The listing builds one solid part. Answer for the finished solid, in the listing's coordinates (mm). A direction names the side the tool comes from. Coordinates: 2 decimals unless noted, no trailing zeros. Write each loop counter-clockwise with the first axis right and the second up, starting at its lowest first coordinate (ties: lowest second). Pieces come first, ordered by that corner, then holes.
from build123d import *

# Parameters (mm, degrees)
SKETCH1_R           = 3.5
SKETCH1_R_2         = 1.8
BOSS_EXTRUDE1_DEPTH = 12
BOSS_EXTRUDE2_DEPTH = 1.5
BOSS_EXTRUDE3_DEPTH = 1.5
CUT_EXTRUDE1_DEPTH  = 5
SKETCH6_R           = 2.75
CUT_EXTRUDE2_DEPTH  = 6
FILLET1_R           = 0.5


with BuildPart() as part:
    # Sketch1 → Boss-Extrude1 (new body)
    with BuildSketch(Plane.XY):
        Circle(SKETCH1_R)
        Circle(SKETCH1_R_2, mode=Mode.SUBTRACT)
    extrude(amount=BOSS_EXTRUDE1_DEPTH)

    # Sketch2 → Boss-Extrude2 (add, symmetric)
    with BuildSketch(Plane(origin=(0, 0, 0), x_dir=(1, 0, 0), z_dir=(0, 1, 0))):
        with BuildLine():
            Line((-5, -17), (-5, -12))
            Line((-5, -12), (5, -12))
            Line((5, -12), (5, -17))
            ThreePointArc((5, -17), (0, -22), (-5, -17))
        make_face()
    extrude(amount=BOSS_EXTRUDE2_DEPTH, both=True)

    # Sketch3 → Boss-Extrude3 (add, symmetric)
    with BuildSketch(Plane(origin=(0, 0, 0), x_dir=(1, 0, 0), z_dir=(0, 1, 0))):
        Polygon((5, -12), (0, -3.339745962), (-5, -12), align=None)
    extrude(amount=BOSS_EXTRUDE3_DEPTH, both=True)

    # Sketch5 → Cut-Extrude1 (cut, symmetric)
    with BuildSketch(Plane(origin=(0, 0, 0), x_dir=(0, 0, -1), z_dir=(1, 0, 0))):
        Polygon((-12, 1.5), (-4, 3.5), (-12, 3.5), align=None)
    cut_extrude1 = extrude(amount=CUT_EXTRUDE1_DEPTH, both=True, mode=Mode.SUBTRACT)

    # Mirror1: Cut-Extrude1 across plane
    add(cut_extrude1.mirror(Plane.ZX), mode=Mode.SUBTRACT)

    # Sketch6 → Cut-Extrude2 (cut, through all)
    with BuildSketch(Plane(origin=(0, 1.5, 0), x_dir=(1, 0, 0), z_dir=(0, 1, 0))):
        with Locations((0, -17)):
            Circle(SKETCH6_R)
    extrude(amount=-CUT_EXTRUDE2_DEPTH, mode=Mode.SUBTRACT)

    # Fillet1
    fillet1_edges = [part.edges().sort_by_distance(p)[0] for p in [
        (-5, -1.5, 14.5),
        (0, -1.5, 22),
        (-5, 1.5, 14.5),
        (5, 1.5, 14.5),
        (-2.342808298, 2.600240235, 7.599039061),
        (2.342808298, -2.600240235, 7.599039061),
        (-4.08113883, 1.5, 10.408485769),
        (-4.08113883, -1.5, 10.408485769),
        (5, -1.5, 14.5),
        (-2.75, -1.5, 17),
        (-2.75, 1.5, 17),
        (4.08113883, 1.5, 10.408485769),
        (0, 1.5, 22),
    ]]
    fillet(fillet1_edges, radius=FILLET1_R)


solid = part.part
1. Flat-ended cylindrical pins translate along their axes: P1, Ø1.5, axis at x = 1, z = 19, coming from the -Y side; P2, Ø4, axis at x = 2.5, y = -2.5, coming from the +Z side; P3, Ø1.5, axis at y = -0.5, z = 2.5, coming from the +X side. Find the tip coordinate at first contact, or state that the pin passes through.
Results found:
P1: stops at y = -1.42
P2: stops at z = 21.87
P3: stops at x = 3.5
2. A tool of negligible diameter and unlimited length cuts with its end or side. For faces 4 (the cylindrical face through (-3.497, 0.154, 4.123)), 5 (the cylindrical face through (4.027, 1.35, 10.599)), from which of +Z, -Z, +X, -X, +Y, -Y can it reach the whole face along a straight path? Write none if from no direction.
Results found:
face 4: -Z
face 5: -Z, +X, +Y
3. Section A-A on y = 0 is taken. Give the vertices of the cut face in (x, z).
Results found:
outline: (-5, 12) - (-3.5, 9.4) - (-3.5, 0) - (-1.8, 0) - (-1.8, 6.46) - (0, 3.34) - (1.8, 6.46) - (1.8, 0) - (3.5, 0) - (3.5, 9.4) - (5, 12) - (5, 17) arc R5 ccw to (-5, 17) - close; hole circle Ø5.5 at (0, 17)
4. Section C-C on z = 8.25 is taken. State how many separate pieces and enclosed holes the cut face has, then the cut area to 3 significant figures.
Results found:
separate pieces: 1
enclosed holes: 2
area: 30.3 mm2
5. For a pull along Z with two mould halves and no side action, classify faces 1 (the cylindrical face through (-0.358, 0.014, 14.273)), 2 (the flat face through (5, 0, 14)), 3 (the cylindrical face through (-4.04, 1.36, 10.64)) as pulls with the +Z half, pulls with the -Z half, needs draft (parallel to the pull), parting line crosses it, or undercut.
Results found:
face 1: undercut
face 2: needs draft
face 3: pulls with the -Z half
6. Find the intervals of material crossed by L1, parallel to X at y = 0, z = 4.5; L2, parallel to X at y = 0.05, z = 17; L3, parallel to Y at x = 0, z = 9.5 (3 decimals), in increasing order.
Results found:
L1: x = -3.5 to -1.8, -0.67 to 0.67, 1.8 to 3.5
L2: x = -5 to -2.75, 2.75 to 5
L3: y = -2.125 to -1.8, -1.5 to 1.5, 1.8 to 2.125
7. Section B-B on z = 13 is taken. Give the vertices of the cut face in (x, y), then the cut area to 3 significant figures.
Results found:
outline: (-5, -1) arc R0.5 ccw to (-4.5, -1.5) - (4.5, -1.5) arc R0.5 ccw to (5, -1) - (5, 1) arc R0.5 ccw to (4.5, 1.5) - (-4.5, 1.5) arc R0.5 ccw to (-5, 1) - close
area: 29.8 mm2
